Can you work these out from the drawing? Everything is in mm from the part's minimum corner. Give positions to 0.01 mm unless a question says otherwise; leave off trailing zeros. Write each loop counter-clockwise with the first axis right and the second up, starting at its lowest first coordinate (ties: lowest second). Pieces come first, ordered by that corner, then holes. Notation, with made-up numbers: (-40, 71.5) - (18, 71.5) arc R35 cw to (18, 108.5) - close; hole circle Ø10 at (26.25, 48). An arc over 180 degrees is marked (long way). Write each question's results on one line, items separated by ' | '. Start each with the question number.
Item 1: Please list where this line runs through material, in increasing order: line 1 along X through (y, z) = (0.95, 0.75).
Item 2: Suppose I cut it at B-B on z = 5.5. List the corners of the cut face in (x, y) for me.
Item 3: Will this pin go through, and if not, where does the flat tip stop? P1, Ø0.6, axis at x = 1, y = 0.5, coming from the +Z side.
Item 4: Suppose I cut it at A-A on y = 0.25. List the corners of the cut face in (x, z) for me, then the cut area to 3 significant figures.
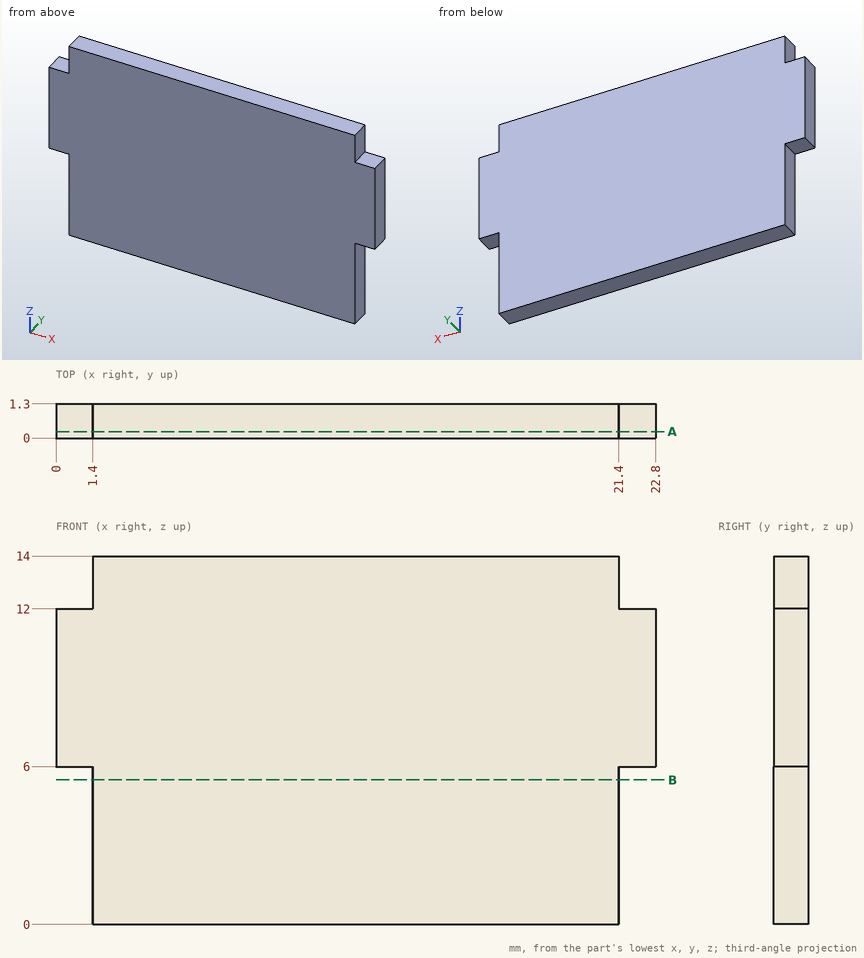
Checked values:
1) line 1: x = 1.4 to 21.4
2) outline: (1.4, 0) - (21.4, 0) - (21.4, 1.3) - (1.4, 1.3) - close
3) P1: stops at z = 12
4) outline: (0, 6) - (1.4, 6) - (1.4, 0) - (21.4, 0) - (21.4, 6) - (22.8, 6) - (22.8, 12) - (21.4, 12) - (21.4, 14) - (1.4, 14) - (1.4, 12) - (0, 12) - close | area: 297 mm^2
